Part model, mm, in its own coordinate system. Face numbers are marked on the shaded views. A direction names the side the tool comes from. Round coordinates to 2 decimals unless told otherwise and drop trailing zeros. Order: outer loops, then holes, each group sorted by start corner. A loop starts at its lowest first (then second) coordinate and runs counter-clockwise, first axis right, second up. Notation, with made-up numbers: (-34, -7.5) -> (-2, -7.5) arc R19 cw to (-2, 29.5) -> close; hole circle Ø7 at (-37, -5.75). An arc over 180 degrees is marked (long way). Answer as a JSON object with one key per item and string values. Group by question number.
Autodesk Inventor part; units mm, degrees
ref_plane "YZ Plane" through (0, 0, 0) normal (1, 0, 0) x (0, 1, 0)
ref_plane "XZ Plane" through (0, 0, 0) normal (0, 1, 0) x (-1, 0, 0)
ref_plane "XY Plane" through (0, 0, 0) normal (0, 0, 1) x (1, 0, 0)
sketch "Sketch1" plane through (0, 0, 0) normal (0, 0, 1) x (1, 0, 0)
  line L0 (0, 48) -> (0, 0)
  line L1 (0, 0) -> (48, 0)
  line L2 (48, 0) -> (48, 3.175)
  line L3 (0, 48) -> (3.175, 48)
  line L4 (3.175, 48) -> (3.175, 3.175)
  line L5 (3.175, 3.175) -> (48, 3.175)
  dimension "d0" = 48
  dimension "d1" = 48
  dimension "d2" = 3.175
  dimension "d3" = 3.175
extrude "Extrusion1" add sketch "Sketch1" along normal mid plane 50.8
sketch "Sketch2" plane through (3.175, 3.175, 25.4) normal (0, 1, 0) x (1, 0, 0)
  line L0 (0, 50.8) -> (0, 0) construction
  line L1 (44.825, 0) -> (0, 0) construction
  line L2 (44.825, 50.8) -> (44.825, 0) construction
  line L3 (0, 50.8) -> (44.825, 50.8) construction
  line L4 (-3.175, 0) -> (44.825, 0)
  line L5 (22.4125, 0) -> (22.4125, 50.8) construction
  line L6 (0, 25.4) -> (44.825, 25.4) construction
  circle A0 centre (22.4125, 25.4) radius 7
  circle A1 centre (14.4125, 33.4) radius 2
  circle A2 centre (11.0988, 25.4) radius 2
  circle A3 centre (14.4125, 17.4) radius 2
  circle A4 centre (22.4125, 14.0863) radius 2
  circle A5 centre (30.4125, 17.4) radius 2
  circle A6 centre (33.7262, 25.4) radius 2
  circle A7 centre (30.4125, 33.4) radius 2
  circle A8 centre (22.4125, 36.7137) radius 2
  circle A9 centre (38.4125, 9.4) radius 2
  circle A10 centre (6.4125, 9.4) radius 2
  circle A11 centre (38.4125, 41.4) radius 2
  circle A12 centre (6.4125, 41.4) radius 2
  point P0 (-3.175, 25.4)
  dimension "d6" = 14
  dimension "d7" = 4
  dimension "d8" = 8
  dimension "d9" = 8
  dimension "d12" = 360
  dimension "d14" = 4
  dimension "d15" = 16
  dimension "d16" = 16
extrude "Extrusion2" cut sketch "Sketch2" against normal through all
sketch "Sketch3" plane through (3.175, 3.175, 25.4) normal (1, 0, 0) x (0, 0, -1)
  line L0 (50.8, 44.825) -> (0, 44.825) construction
  line L1 (0, 0) -> (0, 44.825) construction
  line L2 (50.8, 0) -> (0, 0) construction
  line L3 (50.8, 44.825) -> (50.8, 0) construction
  line L4 (50.8, 44.825) -> (0, 44.825)
  line L5 (25.4, 44.825) -> (25.4, 0) construction
  line L6 (0, 22.4125) -> (50.8, 22.4125) construction
  circle A0 centre (25.4, 22.4125) radius 7
  circle A1 centre (33.4, 30.4125) radius 2
  circle A2 centre (25.4, 33.7262) radius 2
  circle A3 centre (17.4, 30.4125) radius 2
  circle A4 centre (14.0863, 22.4125) radius 2
  circle A5 centre (17.4, 14.4125) radius 2
  circle A6 centre (25.4, 11.0988) radius 2
  circle A7 centre (33.4, 14.4125) radius 2
  circle A8 centre (36.7137, 22.4125) radius 2
  circle A9 centre (9.4, 38.4125) radius 2
  circle A10 centre (9.4, 6.4125) radius 2
  circle A11 centre (41.4, 38.4125) radius 2
  circle A12 centre (41.4, 6.4125) radius 2
  point P0 (25.4, -3.175)
  dimension "d19" = 14
  dimension "d20" = 4
  dimension "d21" = 8
  dimension "d22" = 8
  dimension "d25" = 360
  dimension "d27" = 4
  dimension "d28" = 16
  dimension "d29" = 16
extrude "Extrusion3" cut sketch "Sketch3" against normal through all
chamfer "Chamfer1" distance 2 angle 45 4 edges at (1.5875, 48, 25.4) (1.5875, 48, -25.4) (48, 1.5875, 25.4) (48, 1.5875, -25.4)
properties part number "Arashtrix 48mm x 48mm L-Bracket"
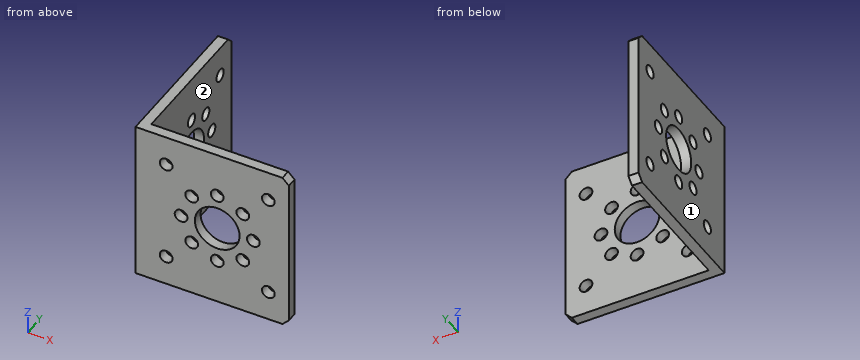
Q1. Wall check: line 1 (Y direction, x = 1, z = 0); line 2 (X direction, y = 1, z = 16). Give the ranges that are in metal, low to high. Write a range as [from, to].
Q2. Which spindle directions (+Z, -Z, +X, -X, +Y, -Y) get a long thin tool onto all of the face, cutting with end or side? Do the marked faces 1 and 2. Say none if no direction does.
Q3. Band-saw the part on A-A (z = 8). List the corners of the cut face in (x, y) (1 decimal), plus the area to 3 significant figures.
Q4. Drop flat-ended pins along their axis: pin 1 Ø5 at (y, z) = (14.27, 0) entering from +X (3 decimals); pin 2 Ø3 at (y, z) = (33.59, 8) entering from +X; pin 3 Ø3 at (x, z) = (24.5, 16) entering from +Y (3 decimals). Give the stop position or say it passes through.
Q5. Band-saw the part on B-B (x = 41). List the corners of the cut face in (y, z) (3 decimals).
Q6. Band-saw the part on D-D (y = 42.5). List the corners of the cut face in (x, z) (3 decimals).
Q7. Band-saw the part on C-C (x = 21.5). List the corners of the cut face in (y, z) (3 decimals), plus the area to 3 significant figures.
Completed:
{
 "1": {"line 1": "[0, 12.27], [16.27, 18.59], [32.59, 34.9], [38.9, 48]", "line 2": "[0, 7.59], [11.59, 39.59], [43.59, 48]"},
 "2": {"face 1": "+Z, -Z, -X, +Y, -Y", "face 2": "+Z, -Z, +X, +Y"},
 "3": {"outline": "(0, 0) -> (15.6, 0) -> (15.6, 3.2) -> (3.2, 3.2) -> (3.2, 15.6) -> (0, 15.6) -> close; (0, 19.6) -> (3.2, 19.6) -> (3.2, 31.6) -> (0, 31.6) -> close; (0, 35.6) -> (3.2, 35.6) -> (3.2, 48) -> (0, 48) -> close; (19.6, 0) -> (31.6, 0) -> (31.6, 3.2) -> (19.6, 3.2) -> close; (35.6, 0) -> (48, 0) -> (48, 3.2) -> (35.6, 3.2) -> close", "area": "244 mm2"},
 "4": {"pin 1": "x = 3.175", "pin 2": "through", "pin 3": "y = 3.175"},
 "5": {"outline": "(0, -25.4) -> (3.175, -25.4) -> (3.175, -17.912) -> (0, -17.912) -> close; (0, -14.088) -> (3.175, -14.088) -> (3.175, 14.088) -> (0, 14.088) -> close; (0, 17.912) -> (3.175, 17.912) -> (3.175, 25.4) -> (0, 25.4) -> close"},
 "6": {"outline": "(0, -25.4) -> (3.175, -25.4) -> (3.175, -17.78) -> (0, -17.78) -> close; (0, -14.22) -> (3.175, -14.22) -> (3.175, 14.22) -> (0, 14.22) -> close; (0, 17.78) -> (3.175, 17.78) -> (3.175, 25.4) -> (0, 25.4) -> close"},
 "7": {"outline": "(0, -25.4) -> (3.175, -25.4) -> (3.175, -5.683) -> (0, -5.683) -> close; (0, 5.683) -> (3.175, 5.683) -> (3.175, 25.4) -> (0, 25.4) -> close", "area": "125 mm2"}
}
